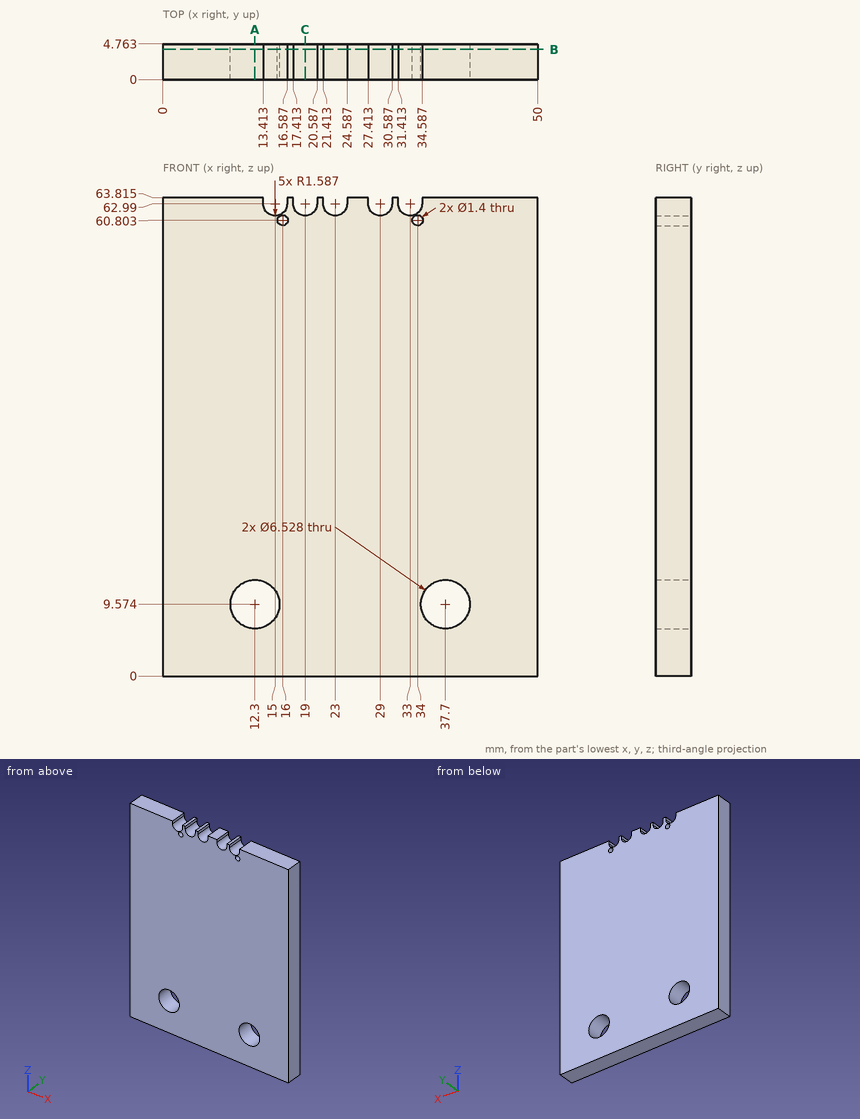
Design review of the part shown in the three views and the two pictorial views. Dimensions are in mm from the part's minimum x, y and z. Coordinates: 2 decimals unless noted, no trailing zeros. Loops run counter-clockwise (first coordinate to the right, second up) from the corner with the lowest first, then second, coordinate; pieces in that order, holes last. Notation, with made-up numbers: (-13, -10.75) - (9, -10.75) arc R32 cw to (9, 25.25) - close; hole circle Ø6 at (-11.5, 63). An arc over 180 degrees is marked (long way). Use a Markdown table: item, result. Add a question column.
Item 1: We need section C-C (x = 19). Give the boundary of the cut face in (y, z).
Item 2: For line 1 (Z direction, x = 38, y = 3) (1 decimal); line 2 (Z direction, x = 39, y = 2.9) (1 decimal), list the stretches that pass through material, from the lowest coordinate up.
Item 3: We need section A-A (x = 12.3). Give the boundary of the cut face in (y, z) (1 decimal).
Item 4: We need section B-B (y = 4.05). Give the boundary of the cut face in (x, z) (1 decimal), and give its area (3 significant figures).
Results list:
| question | item | result |
|---|---|---|
| 1 | outline | (0, 0) - (4.76, 0) - (4.76, 61.4) - (0, 61.4) - close |
| 2 | line 1 | z = 0 to 6.3, 12.8 to 63.8 |
| 2 | line 2 | z = 0 to 6.6, 12.6 to 63.8 |
| 3 | outline | (0, 0) - (4.8, 0) - (4.8, 6.3) - (0, 6.3) - close; (0, 12.8) - (4.8, 12.8) - (4.8, 63.8) - (0, 63.8) - close |
| 4 | outline | (0, 0) - (50, 0) - (50, 63.8) - (34.6, 63.8) - (34.6, 63) arc R1.6 cw to (31.4, 63) - (31.4, 63.8) - (30.6, 63.8) - (30.6, 63) arc R1.6 cw to (27.4, 63) - (27.4, 63.8) - (24.6, 63.8) - (24.6, 63) arc R1.6 cw to (21.4, 63) - (21.4, 63.8) - (20.6, 63.8) - (20.6, 63) arc R1.6 cw to (17.4, 63) - (17.4, 63.8) - (16.6, 63.8) - (16.6, 63) arc R1.6 cw to (13.4, 63) - (13.4, 63.8) - (0, 63.8) - close; hole circle Ø6.5 at (12.3, 9.6); hole circle Ø1.4 at (16, 60.8); hole circle Ø1.4 at (34, 60.8); hole circle Ø6.5 at (37.7, 9.6) |
| 4 | area | 3,090 mm^2 |
